Check sheet for the modelled part. Datum: model origin and axes. Units: mm. A direction names the side the tool comes from. Give positions to 0.01 mm unless a question says otherwise; leave off trailing zeros. Order: outer loops, then holes, each group sorted by start corner. A loop starts at its lowest first (then second) coordinate and runs counter-clockwise, first axis right, second up. Notation, with made-up numbers: (-20, -18) -> (2, -18) arc R27 cw to (2, 18) -> close; hole circle Ø5 at (52.25, -34). An arc over 180 degrees is marked (long way). One line per question, with ' | ' between items. Start each with the question number.
from build123d import *

# Parameters (mm, degrees)
BOSS_EXTRUDE1_DEPTH             = 20
CUT_EXTRUDE3_DEPTH              = 8.5
CUT_EXTRUDE4_REACH              = 107.794
SKETCH5_R                       = 11.5
SKETCH5_R_2                     = 1.6
CUT_EXTRUDE5_REACH              = 109.052
SKETCH6_R                       = 8
SKETCH7_R                       = 3
CUT_EXTRUDE6_DEPTH              = 4
SKETCH8_R                       = 9
CUT_EXTRUDE7_DEPTH              = 6
CUT_EXTRUDE8_START              = -2
SKETCH9_R                       = 9
CUT_EXTRUDE8_DEPTH              = 2
CUT_EXTRUDE9_REACH              = 122.253
CUT_EXTRUDE9_END_RADIUS         = 9
SKETCH10_R                      = 2
FILLET1_R                       = 1
CUT_EXTRUDE10_REACH             = 119.729
SKETCH11_R                      = 2.1
CUT_EXTRUDE10_DIRECTION_2_REACH = 119.729
CUT_EXTRUDE11_REACH             = 127.729
CUT_EXTRUDE11_START             = -8
SKETCH12_R                      = 4
CUT_EXTRUDE12_REACH             = 127.729
CUT_EXTRUDE12_START             = -8
SKETCH13_R                      = 4


with BuildPart() as part:
    # Sketch1 → Boss-Extrude1 (new body)
    with BuildSketch(Plane.XY):
        with BuildLine():
            Line((-50, -15), (50, -15))
            Line((50, -15), (50, -11.808264258))
            ThreePointArc((50, -11.808264258), (49.644862571, -10.16054558), (48.64251158, -8.80541019))
            Line((48.64251158, -8.80541019), (28.393721051, 9.013525475))
            ThreePointArc((28.393721051, 9.013525475), (25.887843573, 12.40136395), (25, 16.520660644))
            Line((25, 16.520660644), (25, 82.520660644))
            ThreePointArc((25, 82.520660644), (22.071067812, 89.591728456), (15, 92.520660644))
            Line((15, 92.520660644), (-15, 92.520660644))
            ThreePointArc((-15, 92.520660644), (-22.071067812, 89.591728456), (-25, 82.520660644))
            Line((-25, 82.520660644), (-25, 16.520660644))
            ThreePointArc((-25, 16.520660644), (-25.887843573, 12.40136395), (-28.393721051, 9.013525475))
            Line((-28.393721051, 9.013525475), (-48.64251158, -8.80541019))
            ThreePointArc((-48.64251158, -8.80541019), (-49.644862571, -10.16054558), (-50, -11.808264258))
            Line((-50, -11.808264258), (-50, -15))
        make_face()
        with BuildLine():
            Line((-19, 10), (19, 10))
            ThreePointArc((19, 10), (19.707106781, 9.707106781), (20, 9))
            Line((20, 9), (20, -9))
            ThreePointArc((20, -9), (19.707106781, -9.707106781), (19, -10))
            Line((19, -10), (-19, -10))
            ThreePointArc((-19, -10), (-19.707106781, -9.707106781), (-20, -9))
            Line((-20, -9), (-20, 9))
            ThreePointArc((-20, 9), (-19.707106781, 9.707106781), (-19, 10))
        make_face(mode=Mode.SUBTRACT)
    extrude(amount=BOSS_EXTRUDE1_DEPTH)

    # Sketch4 → Cut-Extrude3 (cut)
    with BuildSketch(Plane.XY.offset(20)):
        with BuildLine():
            Line((-19.5, 66.5), (19.5, 66.5))
            ThreePointArc((19.5, 66.5), (20.914213562, 65.914213562), (21.5, 64.5))
            Line((21.5, 64.5), (21.5, 25.5))
            ThreePointArc((21.5, 25.5), (20.914213562, 24.085786438), (19.5, 23.5))
            Line((19.5, 23.5), (-19.5, 23.5))
            ThreePointArc((-19.5, 23.5), (-20.914213562, 24.085786438), (-21.5, 25.5))
            Line((-21.5, 25.5), (-21.5, 64.5))
            ThreePointArc((-21.5, 64.5), (-20.914213562, 65.914213562), (-19.5, 66.5))
        make_face()
    extrude(amount=-CUT_EXTRUDE3_DEPTH, mode=Mode.SUBTRACT)

    # Sketch5 → Cut-Extrude4 (cut, up to next)
    with BuildSketch(Plane.XY.offset(11.5), mode=Mode.PRIVATE) as cut_extrude4_sk1:
        with Locations((0, 45)):
            Circle(SKETCH5_R)
    cut_extrude4_tool1 = extrude(cut_extrude4_sk1.sketch, amount=-CUT_EXTRUDE4_REACH, mode=Mode.PRIVATE) & part.part
    # Sketch5 → Cut-Extrude4 (cut, up to next)
    with BuildSketch(Plane.XY.offset(11.5), mode=Mode.PRIVATE) as cut_extrude4_sk2:
        with Locations((-15.75, 60.75)):
            Circle(SKETCH5_R_2)
    cut_extrude4_tool2 = extrude(cut_extrude4_sk2.sketch, amount=-CUT_EXTRUDE4_REACH, mode=Mode.PRIVATE) & part.part
    # Sketch5 → Cut-Extrude4 (cut, up to next)
    with BuildSketch(Plane.XY.offset(11.5), mode=Mode.PRIVATE) as cut_extrude4_sk3:
        with Locations((15.75, 60.75)):
            Circle(SKETCH5_R_2)
    cut_extrude4_tool3 = extrude(cut_extrude4_sk3.sketch, amount=-CUT_EXTRUDE4_REACH, mode=Mode.PRIVATE) & part.part
    # Sketch5 → Cut-Extrude4 (cut, up to next)
    with BuildSketch(Plane.XY.offset(11.5), mode=Mode.PRIVATE) as cut_extrude4_sk4:
        with Locations((-15.75, 29.25)):
            Circle(SKETCH5_R_2)
    cut_extrude4_tool4 = extrude(cut_extrude4_sk4.sketch, amount=-CUT_EXTRUDE4_REACH, mode=Mode.PRIVATE) & part.part
    # Sketch5 → Cut-Extrude4 (cut, up to next)
    with BuildSketch(Plane.XY.offset(11.5), mode=Mode.PRIVATE) as cut_extrude4_sk5:
        with Locations((15.75, 29.25)):
            Circle(SKETCH5_R_2)
    cut_extrude4_tool5 = extrude(cut_extrude4_sk5.sketch, amount=-CUT_EXTRUDE4_REACH, mode=Mode.PRIVATE) & part.part
    add(cut_extrude4_tool1.solids().sort_by_distance((0, 45, 11.5))[0], mode=Mode.SUBTRACT)
    add(cut_extrude4_tool2.solids().sort_by_distance((-15.75, 60.75, 11.5))[0], mode=Mode.SUBTRACT)
    add(cut_extrude4_tool3.solids().sort_by_distance((15.75, 60.75, 11.5))[0], mode=Mode.SUBTRACT)
    add(cut_extrude4_tool4.solids().sort_by_distance((-15.75, 29.25, 11.5))[0], mode=Mode.SUBTRACT)
    add(cut_extrude4_tool5.solids().sort_by_distance((15.75, 29.25, 11.5))[0], mode=Mode.SUBTRACT)

    # Sketch6 → Cut-Extrude5 (cut, up to next)
    with BuildSketch(Plane(origin=(0, 0, 0), x_dir=(-1, 0, 0), z_dir=(0, 0, -1)), mode=Mode.PRIVATE) as cut_extrude5_sk1:
        with Locations((0, 77)):
            Circle(SKETCH6_R)
    cut_extrude5_tool1 = extrude(cut_extrude5_sk1.sketch, amount=-CUT_EXTRUDE5_REACH, mode=Mode.PRIVATE) & part.part
    add(cut_extrude5_tool1.solids().sort_by_distance((0, 77, 0))[0], mode=Mode.SUBTRACT)

    # Sketch7 → Cut-Extrude6 (cut)
    with BuildSketch(Plane(origin=(0, 0, 0), x_dir=(-1, 0, 0), z_dir=(0, 0, -1))):
        with Locations((-15.75, 60.75)):
            Circle(SKETCH7_R)
        with Locations((15.75, 60.75)):
            Circle(SKETCH7_R)
        with Locations((15.75, 29.25)):
            Circle(SKETCH7_R)
        with Locations((-15.75, 29.25)):
            Circle(SKETCH7_R)
    extrude(amount=-CUT_EXTRUDE6_DEPTH, mode=Mode.SUBTRACT)

    # Sketch8 → Cut-Extrude7 (cut)
    with BuildSketch(Plane(origin=(0, 0, 0), x_dir=(-1, 0, 0), z_dir=(0, 0, -1))):
        with Locations((0, 77)):
            Circle(SKETCH8_R)
    extrude(amount=-CUT_EXTRUDE7_DEPTH, mode=Mode.SUBTRACT)

    # Sketch9 → Cut-Extrude8 (cut)
    with BuildSketch(Plane.XY.offset(20).offset(CUT_EXTRUDE8_START)):
        with Locations(Location((0, 77, 0), (0, 0, 180))):
            Circle(SKETCH9_R)
    extrude(amount=CUT_EXTRUDE8_DEPTH, mode=Mode.SUBTRACT)

    # Cut-Extrude9: up to this cylinder (the profile starts outside it)
    cut_extrude9_end = Plane(origin=(0, 77, 3.6), z_dir=(0, 0, -1)) * Cylinder(CUT_EXTRUDE9_END_RADIUS, 263.506, mode=Mode.PRIVATE)
    # Sketch10 → Cut-Extrude9 (cut, up to the surface)
    with BuildSketch(Plane(origin=(0, 92.520660644, 0), x_dir=(1, 0, 0), z_dir=(0, 1, 0)), mode=Mode.PRIVATE) as cut_extrude9_sk1:
        with Locations(Location((0, -3.6, 0), (0, 0, 270))):
            Circle(SKETCH10_R)
    cut_extrude9_tool1 = extrude(cut_extrude9_sk1.sketch, amount=-CUT_EXTRUDE9_REACH, mode=Mode.PRIVATE) - cut_extrude9_end
    add(cut_extrude9_tool1.solids().sort_by_distance((0, 92.520661, 3.6))[0], mode=Mode.SUBTRACT)

    # Fillet1
    fillet1_edges = [part.edges().sort_by_distance(p)[0] for p in [
        (50, -13.404132129, 20),
        (-49.644862571, -10.16054558, 0),
        (-38.518116315, 0.104057643, 0),
        (49.644862571, -10.16054558, 20),
        (-25.887843573, 12.40136395, 0),
        (-25, 49.520660644, 0),
        (-22.071067812, 89.591728456, 0),
        (0, 92.520660644, 0),
        (22.071067812, 89.591728456, 0),
        (25, 49.520660644, 0),
        (25.887843573, 12.40136395, 0),
        (38.518116315, 0.104057643, 20),
        (38.518116315, 0.104057643, 0),
        (49.644862571, -10.16054558, 0),
        (50, -13.404132129, 0),
        (-50, -13.404132129, 0),
        (25.887843573, 12.40136395, 20),
        (25, 49.520660644, 20),
        (22.071067812, 89.591728456, 20),
        (0, 92.520660644, 20),
        (-22.071067812, 89.591728456, 20),
        (-25, 49.520660644, 20),
        (-25.887843573, 12.40136395, 20),
        (-50, -13.404132129, 20),
        (-38.518116315, 0.104057643, 20),
        (-49.644862571, -10.16054558, 20),
    ]]
    fillet(fillet1_edges, radius=FILLET1_R)

    # Sketch11 → Cut-Extrude10 (cut, up to next)
    with BuildSketch(Plane(origin=(-20, 0, 0), x_dir=(0, 0, -1), z_dir=(1, 0, 0)), mode=Mode.PRIVATE) as cut_extrude10_sk1:
        with Locations(Location((-10, 0, 0), (0, 0, 270))):
            Circle(SKETCH11_R)
    cut_extrude10_tool1 = extrude(cut_extrude10_sk1.sketch, amount=-CUT_EXTRUDE10_REACH, mode=Mode.PRIVATE) & part.part
    add(cut_extrude10_tool1.solids().sort_by_distance((-20, 0, 10))[0], mode=Mode.SUBTRACT)

    # Sketch11 → Cut-Extrude10 direction 2 (cut, up to next)
    with BuildSketch(Plane(origin=(-20, 0, 0), x_dir=(0, 0, -1), z_dir=(1, 0, 0)), mode=Mode.PRIVATE) as cut_extrude10_direction_2_sk1:
        with Locations(Location((-10, 0, 0), (0, 0, 270))):
            Circle(SKETCH11_R)
    cut_extrude10_direction_2_tool1 = extrude(cut_extrude10_direction_2_sk1.sketch, amount=CUT_EXTRUDE10_DIRECTION_2_REACH, mode=Mode.PRIVATE) & part.part
    add(cut_extrude10_direction_2_tool1.solids().sort_by_distance((-20, 0, 10))[0], mode=Mode.SUBTRACT)

    # Cut-Extrude11: up to this plane
    cut_extrude11_end = Plane(origin=(-48.64251158, -8.80541019, 20), z_dir=(0.6606278948920247, -0.7507135169227553, 0))
    # Sketch12 → Cut-Extrude11 (cut, up to the surface)
    with BuildSketch(Plane(origin=(-20, 0, 0), x_dir=(0, 0, -1), z_dir=(1, 0, 0)).offset(CUT_EXTRUDE11_START), mode=Mode.PRIVATE) as cut_extrude11_sk1:
        with Locations((-10, 0)):
            Circle(SKETCH12_R)
    cut_extrude11_tool1 = split(extrude(cut_extrude11_sk1.sketch, amount=-CUT_EXTRUDE11_REACH, mode=Mode.PRIVATE), bisect_by=cut_extrude11_end, keep=Keep.BOTH, mode=Mode.PRIVATE)
    add(cut_extrude11_tool1.solids().sort_by_distance((-28, 0, 10))[0], mode=Mode.SUBTRACT)

    # Cut-Extrude12: up to this plane
    cut_extrude12_end = Plane(origin=(48.64251158, -8.80541019, 20), z_dir=(-0.660627894892025, -0.750713516922755, 0))
    # Sketch13 → Cut-Extrude12 (cut, up to the surface)
    with BuildSketch(Plane.ZY.offset(-20).offset(CUT_EXTRUDE12_START), mode=Mode.PRIVATE) as cut_extrude12_sk1:
        with Locations(Location((10, 0, 0), (0, 0, 180))):
            Circle(SKETCH13_R)
    cut_extrude12_tool1 = split(extrude(cut_extrude12_sk1.sketch, amount=-CUT_EXTRUDE12_REACH, mode=Mode.PRIVATE), bisect_by=cut_extrude12_end, keep=Keep.BOTH, mode=Mode.PRIVATE)
    add(cut_extrude12_tool1.solids().sort_by_distance((28, 0, 10))[0], mode=Mode.SUBTRACT)


solid = part.part
1. Cross-section at A-A on x = 0. Give the number of separate pieces and of enclosed holes in the cut face, and give its area (3 significant figures).
2. Mould release check, pull along X, two halves, no side actions. Record for faces 1 (the face through (-25, 50, 10)), 2 (the face through (0, 92.521, 10)), 3 (the face through (-13.54, 62.78, 1.97)): +X half, -X half, draft (parallel to the pull), parting line (faces both ways), or undercut.
3. Scan lines: probe 1 along Y at (x, z) = (-13.5, 11.75); probe 2 along Y at (x, z) = (-15.5, 8); probe 3 along Y at (x, z) = (15.75, 2.4). Record each from-to range of solid material in increasing order.
4. Cross-section at B-B on y = 60.75. Record the boundary of the cut face in (x, z), and give its area (3 significant figures).
5. Go/stop test with flat-tipped pins: pin 1 (1.5 mm diameter, centred on x = 21, z = 11, fed in from +Y); pin 2 (1.5 mm diameter, centred on y = 1, z = 11, fed in from +X); pin 3 (10 mm diameter, centred on x = 36, z = 12.5, fed in from +Y). Record where each tip stops, or that it passes through.
6. Cross-section at C-C on y = 48. Record the boundary of the cut face in (x, z), and give its area (3 significant figures).
7. Tool access check on faces 4 (the face through (1.951, 68.214, 2.958)), 5 (the face through (1.951, 85.786, 18.986)), 6 (the face through (-33.839, -3.905, 10.867)), 7 (the face through (-15.958, 62.336, 7.802)). Record the directions out of +Z, -Z, +X, -X, +Y, -Y that give a thin tool (end or side, any length) a straight path to the whole face; none if there is none.
Response values:
1) separate pieces: 5 | enclosed holes: 0 | area: 758 mm²
2) face 1: -X half | face 2: draft | face 3: undercut
3) probe 1: y = -15 to -10, 10 to 23.5, 66.5 to 92.52 | probe 2: y = -15 to -10, 10 to 27.67, 30.83 to 59.17, 62.33 to 92.51 | probe 3: y = -15 to -10, 10 to 26.25, 32.25 to 57.75, 63.75 to 92.49
4) outline: (-25, 1) arc R1 ccw to (-24, 0) -> (-18.75, 0) -> (-18.75, 4) -> (-17.35, 4) -> (-17.35, 11.5) -> (-21.5, 11.5) -> (-21.5, 20) -> (-24, 20) arc R1 ccw to (-25, 19) -> close; (-14.15, 4) -> (-12.75, 4) -> (-12.75, 0) -> (12.75, 0) -> (12.75, 4) -> (14.15, 4) -> (14.15, 11.5) -> (-14.15, 11.5) -> close; (17.35, 4) -> (18.75, 4) -> (18.75, 0) -> (24, 0) arc R1 ccw to (25, 1) -> (25, 19) arc R1 ccw to (24, 20) -> (21.5, 20) -> (21.5, 11.5) -> (17.35, 11.5) -> close | area: 538 mm²
5) pin 1: stops at y = 91.03 | pin 2: stops at x = 28 | pin 3: stops at y = 6.72
6) outline: (-25, 1) arc R1 ccw to (-24, 0) -> (-11.1, 0) -> (-11.1, 11.5) -> (-21.5, 11.5) -> (-21.5, 20) -> (-24, 20) arc R1 ccw to (-25, 19) -> close; (11.1, 0) -> (24, 0) arc R1 ccw to (25, 1) -> (25, 19) arc R1 ccw to (24, 20) -> (21.5, 20) -> (21.5, 11.5) -> (11.1, 11.5) -> close | area: 378 mm²
7) face 4: -Z | face 5: +Z | face 6: -X | face 7: +Z, -Z
